```python
from build123d import *

# Parameters (mm, degrees)
SKETCH1_W                 = 130
SKETCH1_H                 = 125
BOSS_EXTRUDE1_DEPTH       = 5
SKETCH2_R                 = 1.5
SKETCH2_R_2               = 12.65
CUT_EXTRUDE1_DEPTH        = 10
SKETCH4_R                 = 1.5
CUT_EXTRUDE3_DEPTH        = 10
BOSS_EXTRUDE2_DEPTH       = 2
MIRROR7_COPY_1_SKETCH_R   = 1.5
MIRROR7_COPY_1_SKETCH_R_2 = 12.65
MIRROR7_COPY_1_DEPTH      = 10
MIRROR7_COPY_2_DEPTH      = 2
SKETCH10_R                = 1.5
CUT_EXTRUDE8_DEPTH        = 91.311959341
SKETCH11_R                = 2.65
CUT_EXTRUDE9_DEPTH        = 0.5
CUT_EXTRUDE10_DEPTH       = 91.444734507
CUT_EXTRUDE11_DEPTH       = 91.444734507
CUT_EXTRUDE12_DEPTH       = 91.444734507
SKETCH15_W                = 130
SKETCH15_H                = 125
SKETCH15_W_2              = 5
SKETCH15_H_2              = 5
CUT_EXTRUDE14_DEPTH       = 2
CUT_EXTRUDE15_START       = -8
SKETCH17_W                = 137.629855092
SKETCH17_H                = 131.076052468
CUT_EXTRUDE15_DEPTH       = 2
SKETCH18_W                = 13.527386212
SKETCH18_H                = 6.370278614
CUT_EXTRUDE16_DEPTH       = 1
SKETCH19_R                = 1
CUT_EXTRUDE17_DEPTH       = 5
SKETCH20_W                = 6.657761804
SKETCH20_H                = 4.4233075
CUT_EXTRUDE18_DEPTH       = 2


with BuildPart() as part:
    # Sketch1 → Boss-Extrude1 (new body)
    with BuildSketch(Plane(origin=(0, 0, 0), x_dir=(1, 0, 0), z_dir=(0, 1, 0))):
        Rectangle(SKETCH1_W, SKETCH1_H)
    extrude(amount=BOSS_EXTRUDE1_DEPTH)

    # Sketch2 → Cut-Extrude1 (cut)
    with BuildSketch(Plane(origin=(0, 5, 0), x_dir=(1, 0, 0), z_dir=(0, 1, 0))):
        with Locations(Location((-61, -52.5, 0), (0, 0, 270))):
            Circle(SKETCH2_R)
        with Locations(Location((-36, -52.5, 0), (0, 0, 270))):
            Circle(SKETCH2_R)
        with Locations(Location((-36, -10.5, 0), (0, 0, 270))):
            Circle(SKETCH2_R)
        with Locations(Location((-61, -10.5, 0), (0, 0, 270))):
            Circle(SKETCH2_R)
        with Locations(Location((-45.5, -31.5, 0), (0, 0, 270))):
            Circle(SKETCH2_R_2)
    cut_extrude1 = extrude(amount=-CUT_EXTRUDE1_DEPTH, mode=Mode.SUBTRACT)

    # Mirror3: Cut-Extrude1 across plane
    add(cut_extrude1.mirror(Plane.ZY), mode=Mode.SUBTRACT)

    # Sketch4 → Cut-Extrude3 (cut)
    with BuildSketch(Plane(origin=(0, 5, 0), x_dir=(1, 0, 0), z_dir=(0, 1, 0))):
        with Locations(Location((0, 47.5, 0), (0, 0, 270))):
            Circle(SKETCH4_R)
        with Locations(Location((12.049810205, 55, 0), (0, 0, 270))):
            Circle(SKETCH4_R)
        with Locations(Location((-12.049810205, 55, 0), (0, 0, 270))):
            Circle(SKETCH4_R)
    extrude(amount=-CUT_EXTRUDE3_DEPTH, mode=Mode.SUBTRACT)

    # Sketch5 → Boss-Extrude2 (add)
    with BuildSketch(Plane.XZ):
        Polygon((-65, 58.6), (-65, 56.6), (-31.8, 56.6), (-31.8, 6.4), (-65, 6.4), (-65, 4.4), (-29.8, 4.4), (-29.8, 58.6), align=None)
    boss_extrude2 = extrude(amount=BOSS_EXTRUDE2_DEPTH)

    # Mirror5: Boss-Extrude2 across plane
    add(boss_extrude2.mirror(Plane.ZY))

    # Mirror7: Cut-Extrude1, Boss-Extrude2 across plane
    add(cut_extrude1.mirror(Plane.XY.offset(-1.9)), mode=Mode.SUBTRACT)
    add(boss_extrude2.mirror(Plane.XY.offset(-1.9)))

    # Mirror7 copy 1 sketch → Mirror7 copy 1 (cut)
    with BuildSketch(Plane(origin=(0, 5, -3.8), x_dir=(-1, 0, 0), z_dir=(0, 1, 0))):
        with Locations(Location((-61, -52.5, 0), (0, 0, 270))):
            Circle(MIRROR7_COPY_1_SKETCH_R)
        with Locations(Location((-36, -52.5, 0), (0, 0, 270))):
            Circle(MIRROR7_COPY_1_SKETCH_R)
        with Locations(Location((-36, -10.5, 0), (0, 0, 270))):
            Circle(MIRROR7_COPY_1_SKETCH_R)
        with Locations(Location((-61, -10.5, 0), (0, 0, 270))):
            Circle(MIRROR7_COPY_1_SKETCH_R)
        with Locations(Location((-45.5, -31.5, 0), (0, 0, 270))):
            Circle(MIRROR7_COPY_1_SKETCH_R_2)
    extrude(amount=-MIRROR7_COPY_1_DEPTH, mode=Mode.SUBTRACT)

    # Mirror7 copy 2 sketch → Mirror7 copy 2 (add)
    with BuildSketch(Plane(origin=(0, 0, -3.8), x_dir=(-1, 0, 0), z_dir=(0, -1, 0))):
        Polygon((-65, 58.6), (-65, 56.6), (-31.8, 56.6), (-31.8, 6.4), (-65, 6.4), (-65, 4.4), (-29.8, 4.4), (-29.8, 58.6), align=None)
    extrude(amount=MIRROR7_COPY_2_DEPTH)

    # Sketch10 → Cut-Extrude8 (cut, through all)
    with BuildSketch(Plane(origin=(0, 0, 0), x_dir=(-1, 0, 0), z_dir=(0, -1, 0))):
        with Locations(Location((-24.17, -42.03, 0), (0, 0, 90))):
            Circle(SKETCH10_R)
        with Locations(Location((24.17, -42.03, 0), (0, 0, 90))):
            Circle(SKETCH10_R)
        with Locations(Location((-8.73, 9.6, 0), (0, 0, 90))):
            Circle(SKETCH10_R)
        with Locations(Location((19.29, 9.6, 0), (0, 0, 90))):
            Circle(SKETCH10_R)
        with Locations(Location((-24.17, 33.11, 0), (0, 0, 90))):
            Circle(SKETCH10_R)
        with Locations(Location((24.17, 40.6, 0), (0, 0, 90))):
            Circle(SKETCH10_R)
    extrude(amount=-CUT_EXTRUDE8_DEPTH, mode=Mode.SUBTRACT)

    # Sketch11 → Cut-Extrude9 (cut)
    with BuildSketch(Plane.XZ):
        with Locations(Location((-12.049810205, -55, 0), (0, 0, 270))):
            Circle(SKETCH11_R)
        with Locations(Location((0, -47.5, 0), (0, 0, 270))):
            Circle(SKETCH11_R)
        with Locations(Location((12.049810205, -55, 0), (0, 0, 270))):
            Circle(SKETCH11_R)
        with Locations(Location((-24.17, -40.6, 0), (0, 0, 270))):
            Circle(SKETCH11_R)
        with Locations(Location((24.17, -33.11, 0), (0, 0, 270))):
            Circle(SKETCH11_R)
        with Locations(Location((8.73, -9.6, 0), (0, 0, 270))):
            Circle(SKETCH11_R)
        with Locations(Location((-19.29, -9.6, 0), (0, 0, 270))):
            Circle(SKETCH11_R)
        with Locations(Location((-24.17, 42.03, 0), (0, 0, 270))):
            Circle(SKETCH11_R)
        with Locations(Location((24.17, 42.03, 0), (0, 0, 270))):
            Circle(SKETCH11_R)
        with Locations(Location((-61, -14.3, 0), (0, 0, 270))):
            Circle(SKETCH11_R)
        with Locations(Location((-36, -14.3, 0), (0, 0, 270))):
            Circle(SKETCH11_R)
        with Locations(Location((-61, -56.3, 0), (0, 0, 270))):
            Circle(SKETCH11_R)
        with Locations(Location((-36, -56.3, 0), (0, 0, 270))):
            Circle(SKETCH11_R)
        with Locations(Location((36, -56.3, 0), (0, 0, 270))):
            Circle(SKETCH11_R)
        with Locations(Location((61, -56.3, 0), (0, 0, 270))):
            Circle(SKETCH11_R)
        with Locations(Location((36, -14.3, 0), (0, 0, 270))):
            Circle(SKETCH11_R)
        with Locations(Location((61, -14.3, 0), (0, 0, 270))):
            Circle(SKETCH11_R)
        with Locations(Location((36, 10.5, 0), (0, 0, 270))):
            Circle(SKETCH11_R)
        with Locations(Location((61, 10.5, 0), (0, 0, 270))):
            Circle(SKETCH11_R)
        with Locations(Location((61, 52.5, 0), (0, 0, 270))):
            Circle(SKETCH11_R)
        with Locations(Location((36, 52.5, 0), (0, 0, 270))):
            Circle(SKETCH11_R)
        with Locations(Location((-36, 52.5, 0), (0, 0, 270))):
            Circle(SKETCH11_R)
        with Locations(Location((-36, 10.5, 0), (0, 0, 270))):
            Circle(SKETCH11_R)
        with Locations(Location((-61, 10.5, 0), (0, 0, 270))):
            Circle(SKETCH11_R)
        with Locations(Location((-61, 52.5, 0), (0, 0, 270))):
            Circle(SKETCH11_R)
    extrude(amount=-CUT_EXTRUDE9_DEPTH, mode=Mode.SUBTRACT)

    # Sketch12 → Cut-Extrude10 (cut, through all)
    with BuildSketch(Plane(origin=(0, 5, 0), x_dir=(1, 0, 0), z_dir=(0, 1, 0))):
        Polygon((-2.363095604, -26.45), (-20.17, 1.845056316), (-20.17, -54.745056316), align=None)
        Polygon((17.806904396, 5.6), (-17.806904396, 5.6), (0, -22.695056316), align=None)
        Polygon((20.17, -54.745056316), (20.17, 1.845056316), (2.363095604, -26.45), align=None)
        Polygon((0, -30.204943684), (-17.806904396, -58.5), (17.806904396, -58.5), align=None)
    extrude(amount=-CUT_EXTRUDE10_DEPTH, mode=Mode.SUBTRACT)

    # Sketch13 → Cut-Extrude11 (cut, through all)
    with BuildSketch(Plane(origin=(0, 5, 0), x_dir=(1, 0, 0), z_dir=(0, 1, 0))):
        Polygon((-61, 1.9), (-61, -3.1), (-24.17, -3.1), (-24.17, 6.9), (-61, 6.9), align=None)
    cut_extrude11 = extrude(amount=-CUT_EXTRUDE11_DEPTH, mode=Mode.SUBTRACT)

    # Mirror9: Cut-Extrude11 across plane
    add(cut_extrude11.mirror(Plane.ZY), mode=Mode.SUBTRACT)

    # Sketch14 → Cut-Extrude12 (cut, through all)
    with BuildSketch(Plane(origin=(0, 5, 0), x_dir=(1, 0, 0), z_dir=(0, 1, 0))):
        Polygon((-3.110442245, 28.55), (-17.806904396, 40.888590935), (-17.806904396, 16.211409065), align=None)
        Polygon((14.696462151, 43.5), (-14.696462151, 43.5), (0, 31.161409065), align=None)
        Polygon((17.806904396, 16.211409065), (17.806904396, 40.888590935), (3.110442245, 28.55), align=None)
        Polygon((0, 25.938590935), (-14.696462151, 13.6), (14.696462151, 13.6), align=None)
    extrude(amount=-CUT_EXTRUDE12_DEPTH, mode=Mode.SUBTRACT)

    # Sketch15 → Cut-Extrude14 (cut)
    with BuildSketch(Plane(origin=(0, 5, 0), x_dir=(1, 0, 0), z_dir=(0, 1, 0))):
        Rectangle(SKETCH15_W, SKETCH15_H)
        with Locations((-61, 56.3)):
            Rectangle(SKETCH15_W_2, SKETCH15_H_2, mode=Mode.SUBTRACT)
        with Locations((-36, 56.3)):
            Rectangle(SKETCH15_W_2, SKETCH15_H_2, mode=Mode.SUBTRACT)
        with Locations((-12.049810205, 55)):
            Rectangle(SKETCH15_W_2, SKETCH15_H_2, mode=Mode.SUBTRACT)
        with Locations((0, 47.5)):
            Rectangle(SKETCH15_W_2, SKETCH15_H_2, mode=Mode.SUBTRACT)
        with Locations((12.049810205, 55)):
            Rectangle(SKETCH15_W_2, SKETCH15_H_2, mode=Mode.SUBTRACT)
        with Locations((36, 56.3)):
            Rectangle(SKETCH15_W_2, SKETCH15_H_2, mode=Mode.SUBTRACT)
        with Locations((61, 56.3)):
            Rectangle(SKETCH15_W_2, SKETCH15_H_2, mode=Mode.SUBTRACT)
        with Locations((36, 14.3)):
            Rectangle(SKETCH15_W_2, SKETCH15_H_2, mode=Mode.SUBTRACT)
        with Locations((61, 14.3)):
            Rectangle(SKETCH15_W_2, SKETCH15_H_2, mode=Mode.SUBTRACT)
        with Locations((24.17, 33.11)):
            Rectangle(SKETCH15_W_2, SKETCH15_H_2, mode=Mode.SUBTRACT)
        with Locations((36, -10.5)):
            Rectangle(SKETCH15_W_2, SKETCH15_H_2, mode=Mode.SUBTRACT)
        with Locations((61, -10.5)):
            Rectangle(SKETCH15_W_2, SKETCH15_H_2, mode=Mode.SUBTRACT)
        with Locations((24.17, -42.03)):
            Rectangle(SKETCH15_W_2, SKETCH15_H_2, mode=Mode.SUBTRACT)
        with Locations((36, -52.5)):
            Rectangle(SKETCH15_W_2, SKETCH15_H_2, mode=Mode.SUBTRACT)
        with Locations((61, -52.5)):
            Rectangle(SKETCH15_W_2, SKETCH15_H_2, mode=Mode.SUBTRACT)
        with Locations((-24.17, -42.03)):
            Rectangle(SKETCH15_W_2, SKETCH15_H_2, mode=Mode.SUBTRACT)
        with Locations((-36, -52.5)):
            Rectangle(SKETCH15_W_2, SKETCH15_H_2, mode=Mode.SUBTRACT)
        with Locations((-36, -10.5)):
            Rectangle(SKETCH15_W_2, SKETCH15_H_2, mode=Mode.SUBTRACT)
        with Locations((8.73, 9.6)):
            Rectangle(SKETCH15_W_2, SKETCH15_H_2, mode=Mode.SUBTRACT)
        with Locations((-19.29, 9.6)):
            Rectangle(SKETCH15_W_2, SKETCH15_H_2, mode=Mode.SUBTRACT)
        with Locations((-24.17, 40.6)):
            Rectangle(SKETCH15_W_2, SKETCH15_H_2, mode=Mode.SUBTRACT)
        with Locations((-61, 14.3)):
            Rectangle(SKETCH15_W_2, SKETCH15_H_2, mode=Mode.SUBTRACT)
        with Locations((-36, 14.3)):
            Rectangle(SKETCH15_W_2, SKETCH15_H_2, mode=Mode.SUBTRACT)
        with Locations((-61, -10.5)):
            Rectangle(SKETCH15_W_2, SKETCH15_H_2, mode=Mode.SUBTRACT)
        with Locations((-61, -52.5)):
            Rectangle(SKETCH15_W_2, SKETCH15_H_2, mode=Mode.SUBTRACT)
    extrude(amount=-CUT_EXTRUDE14_DEPTH, mode=Mode.SUBTRACT)

    # Sketch17 → Cut-Extrude15 (cut)
    with BuildSketch(Plane(origin=(0, 13, 0), x_dir=(1, 0, 0), z_dir=(0, 1, 0)).offset(CUT_EXTRUDE15_START)):
        with Locations((0.756207995, -1.260346658)):
            Rectangle(SKETCH17_W, SKETCH17_H)
    extrude(amount=-CUT_EXTRUDE15_DEPTH, mode=Mode.SUBTRACT)

    # Sketch18 → Cut-Extrude16 (cut)
    with BuildSketch(Plane(origin=(0, 3, 0), x_dir=(1, 0, 0), z_dir=(0, 1, 0))):
        with Locations((-26.648289701, -59.314860693)):
            Rectangle(SKETCH18_W, SKETCH18_H)
    extrude(amount=-CUT_EXTRUDE16_DEPTH, mode=Mode.SUBTRACT)

    # Sketch19 → Cut-Extrude17 (cut)
    with BuildSketch(Plane(origin=(0, 2, 0), x_dir=(1, 0, 0), z_dir=(0, 1, 0))):
        with Locations(Location((-23.4201, -57.55, 0), (0, 0, 270))):
            Circle(SKETCH19_R)
        with Locations(Location((-29.9201, -57.55, 0), (0, 0, 270))):
            Circle(SKETCH19_R)
    extrude(amount=-CUT_EXTRUDE17_DEPTH, mode=Mode.SUBTRACT)

    # Sketch20 → Cut-Extrude18 (cut)
    with BuildSketch(Plane.XZ):
        with Locations((-29.482363252, 57.493891291)):
            Rectangle(SKETCH20_W, SKETCH20_H)
    extrude(amount=CUT_EXTRUDE18_DEPTH, mode=Mode.SUBTRACT)


solid = part.part
```
Here's how the part is built. I have some questions about the finished solid (model axes, mm). A direction names the side the tool comes from. Coordinates: 2 decimals unless noted, no trailing zeros. Write each loop counter-clockwise with the first axis right and the second up, starting at its lowest first coordinate (ties: lowest second). Pieces come first, ordered by that corner, then holes. Notation, with made-up numbers: (-0.5, 4) -> (13.5, 4) arc R19 cw to (13.5, 35) -> close; hole circle Ø4 at (61.25, -25). An arc over 180 degrees is marked (long way). Use a Markdown table: item, result. Add a question column.
(1) For faces 4 (the cylindrical face through (0.117, 0.246, -44.853)), 5 (the flat face through (10.562, 1.521, -34.806)), which set-ups out of +Z, -Z, +X, -X, +Y, -Y let a thin tool reach every point of the face, with its end or its side?
(2) I'm going to push flat-ended pins straight in: P1, Ø6, axis at x = -61, z = -56.3, coming from the -Y side; P2, Ø2.5, axis at x = 23.5, z = 41.5, coming from the -Y side; P3, Ø1.6, axis at x = -42.5, y = -1, coming from the +Z side. Where does each tip first touch, or does it pass through?
(3) If we section it at A-A, the plane x = -45.5: State how many separate pieces and enclosed holes the cut face has, and give its area (3 significant figures).
(4) If we section it at B-B, the plane z = 17: Write out the boundary of the cut face in (x, y), and give its area (3 significant figures).
(5) We'd pull the mould along X, two halves only. Please class faces 1 (the flat face through (-1, 0.5, -49)), 2 (the flat face through (59, 0, 31)), 3 (the flat face through (60, 0.5, 51)): +X half, -X half, draft (parallel to the pull), parting line (faces both ways), or undercut.
(6) Please list where these lines run through material, in increasing order: line 1 (Z direction, x = -49.5, y = -1.8); line 2 (Z direction, x = 38.5, y = 2.55); line 3 (Z direction, x = 31.5, y = -1.5).
Outcome:
| question | item | result |
|---|---|---|
| 1 | face 4 | -Y |
| 1 | face 5 | +Y, -Y |
| 2 | P1 | stops at y = 0 |
| 2 | P2 | stops at y = 0.5 |
| 2 | P3 | stops at z = 58.6 |
| 3 | separate pieces | 4 |
| 3 | enclosed holes | 0 |
| 3 | area | 209 mm^2 |
| 4 | outline | (-65, 0) -> (-31.8, 0) -> (-31.8, -2) -> (-29.8, -2) -> (-29.8, 0) -> (-20.17, 0) -> (-20.17, 3) -> (-65, 3) -> close; (-8.31, 0) -> (-3.58, 0) -> (-3.58, 3) -> (-8.31, 3) -> close; (3.58, 0) -> (8.31, 0) -> (8.31, 3) -> (3.58, 3) -> close; (20.17, 0) -> (29.8, 0) -> (29.8, -2) -> (31.8, -2) -> (31.8, 0) -> (65, 0) -> (65, 3) -> (20.17, 3) -> close |
| 4 | area | 305 mm^2 |
| 5 | face 1 | undercut |
| 5 | face 2 | draft |
| 5 | face 3 | undercut |
| 6 | line 1 | z = -62.4 to -60.4, -10.2 to -8.2, 4.4 to 6.4, 56.6 to 58.6 |
| 6 | line 2 | z = -62.5 to -45.84, -24.76 to -6.9, 3.1 to 20.96, 42.04 to 62.5 |
| 6 | line 3 | z = -62.4 to -8.2, 4.4 to 58.6 |
